Geometry: final body of the model. Coordinates: model frame, mm. A direction names the side the tool comes from. Coordinates: 2 decimals unless noted, no trailing zeros. Order: outer loops, then holes, each group sorted by start corner. A loop starts at its lowest first (then second) coordinate and runs counter-clockwise, first axis right, second up. Notation, with made-up numbers: (-39, 12.5) - (15, 12.5) arc R8 cw to (15, 20.5) - close; hole circle Ø8 at (16, -12). An arc over 180 degrees is marked (long way). Use a Markdown table: item, result. Add a question column.
```python
from build123d import *

# Parameters (mm, degrees)
SKETCH1_W                    = 83.185
SKETCH1_H                    = 41.91
SKETCH1_R                    = 2.54
SKETCH1_W_2                  = 57.15
SKETCH1_H_2                  = 25.4
ROVER_MOUNT_DEPTH            = 2.54
SIDE_WALLS_REACH             = 85.531
SIDE_WALLS_DIRECTION_2_DEPTH = 6.000000034
BACK_BRACES_DEPTH            = 2.54
FRONT_COVER_DEPTH            = 2.54
SKETCH5_W                    = 83.185
SKETCH5_H                    = 6.000000034
CLEANUP_DEPTH                = 31.75
FILLET1_R                    = 3.81
FILLET2_R                    = 6.35


with BuildPart() as part:
    # Sketch1 → Rover mount (new body)
    with BuildSketch(Plane.XY):
        with Locations((33.3375, -15.875)):
            Rectangle(SKETCH1_W, SKETCH1_H)
        with Locations((66.675, -31.75)):
            Circle(SKETCH1_R, mode=Mode.SUBTRACT)
        with Locations((69.85, 0)):
            Circle(SKETCH1_R, mode=Mode.SUBTRACT)
        with Locations((-3.175, -31.75)):
            Circle(SKETCH1_R, mode=Mode.SUBTRACT)
        Circle(SKETCH1_R, mode=Mode.SUBTRACT)
        with Locations((33.3375, -15.875)):
            Rectangle(SKETCH1_W_2, SKETCH1_H_2, mode=Mode.SUBTRACT)
    extrude(amount=ROVER_MOUNT_DEPTH)

    # Side Walls: up to this face of the body (flat: up to its plane)
    side_walls_end = Plane(part.part.faces().sort_by_distance((73.998539194, -15.875, 0))[0])
    # Sketch2 → Side Walls (add, up to the picked face)
    with BuildSketch(Plane.XY.offset(2.54), mode=Mode.PRIVATE) as side_walls_sk1:
        Polygon((-50.6625, -68.58), (-8.255, -68.58), (-8.255, -36.83), (4.445, -36.83), (4.445, -68.58), (62.23, -68.58), (62.23, -36.83), (74.93, -36.83), (74.93, -68.58), (117.3375, -68.58), (117.3375, 36.42), (122.4175, 36.42), (122.4175, -72.39), (-55.7425, -72.39), (-55.7425, 36.42), (-50.6625, 36.42), align=None)
    side_walls_tool1 = split(extrude(side_walls_sk1.sketch, amount=-SIDE_WALLS_REACH, mode=Mode.PRIVATE), bisect_by=side_walls_end, keep=Keep.BOTH, mode=Mode.PRIVATE)
    add(side_walls_tool1.solids().sort_by(Axis((-29.45875, -70.667597, 2.54), (0, 0, -1)))[0])

    # Sketch2 → Side Walls direction 2 (add)
    with BuildSketch(Plane.XY.offset(2.54)):
        Polygon((-50.6625, -68.58), (-8.255, -68.58), (-8.255, -36.83), (4.445, -36.83), (4.445, -68.58), (62.23, -68.58), (62.23, -36.83), (74.93, -36.83), (74.93, -68.58), (117.3375, -68.58), (117.3375, 36.42), (122.4175, 36.42), (122.4175, -72.39), (-55.7425, -72.39), (-55.7425, 36.42), (-50.6625, 36.42), align=None)
    extrude(amount=SIDE_WALLS_DIRECTION_2_DEPTH)

    # Sketch3 → Back Braces (add)
    with BuildSketch(Plane.XY.offset(2.54)):
        Polygon((-12.779899069, 1.716266635), (-55.7425, -68.58), (-49.3925, -68.58), (-8.255, -1.27), (-8.255, 5.08), (-55.7425, 36.42), (-55.7425, 30.07), align=None)
        Polygon((79.454899069, 1.716266635), (122.4175, -68.58), (116.0675, -68.58), (74.93, -1.27), (74.93, 5.08), (122.4175, 36.42), (122.4175, 30.07), align=None)
    extrude(amount=-BACK_BRACES_DEPTH)

    # Sketch4 → Front Cover (add)
    with BuildSketch(Plane.XY.offset(8.540000034)):
        Polygon((-55.7425, 36.42), (-45.5825, 36.42), (-45.5825, -63.5), (112.2575, -63.5), (112.2575, 36.42), (122.4175, 36.42), (122.4175, -72.39), (-55.7425, -72.39), align=None)
    extrude(amount=FRONT_COVER_DEPTH)

    # Sketch5 → Cleanup (cut)
    with BuildSketch(Plane(origin=(0, -36.83, 0), x_dir=(1, 0, 0), z_dir=(0, 1, 0))):
        with Locations((33.3375, -5.540000017)):
            Rectangle(SKETCH5_W, SKETCH5_H)
    extrude(amount=-CLEANUP_DEPTH, mode=Mode.SUBTRACT)

    # Fillet1
    fillet1_edges = [part.edges().sort_by_distance(p)[0] for p in [
        (117.3375, 26.717387207, 1.27),
        (117.3375, 33.067387207, 1.27),
        (117.3375, -60.268002431, 1.27),
        (79.454899069, 1.716266635, 1.27),
        (116.0675, -68.58, 1.27),
        (74.93, -1.27, 1.27),
        (-8.255, -68.58, 1.27),
        (4.445, -68.58, 1.27),
        (62.23, -68.58, 1.27),
        (74.93, -68.58, 1.27),
        (-8.255, 5.08, 1.27),
        (74.93, 5.08, 1.27),
        (-49.3925, -68.58, 1.27),
        (-12.779899069, 1.716266635, 1.27),
        (-50.6625, 33.067387207, 1.27),
        (-8.255, -1.27, 1.27),
        (-50.6625, -60.268002431, 1.27),
        (-50.6625, 26.717387207, 1.27),
    ]]
    fillet(fillet1_edges, radius=FILLET1_R)

    # Fillet2
    fillet2_edges = [part.edges().sort_by_distance(p)[0] for p in [
        (4.7625, -3.175, 1.27),
        (4.7625, -28.575, 1.27),
        (61.9125, -28.575, 1.27),
        (61.9125, -3.175, 1.27),
    ]]
    fillet(fillet2_edges, radius=FILLET2_R)


solid = part.part
```
1) Set-up query: faces 1 (the face through (34, -66, 8.54)), 2 (the face through (-45.95, -66.58, 1.25)), 3 (the face through (-30.797, -38.153, 1.288)). Return all of +Z, -Z, +X, -X, +Y, -Y with unobstructed straight access to the full face (end or side cutting, diameter ignored); none if empty.
2) Section B-B (x = 22.5). Return loops of the section in (y, z) (3 decimals), then the cut area to 3 significant figures.
3) Section D-D (y = -31.75). Give the number of separate pieces and of enclosed holes in the cut face, then the cut area to 3 significant figures.
4) Pin query (flat end, axial travel): pin 1 (2 mm diameter, centred on x = 40.5, z = 1.5, fed in from +Y); pin 2 (2.5 mm diameter, centred on x = -7.5, z = 5.5, fed in from +Y). Return the tip coordinate at first contact, or that it passes through.
5) Draft query along Z for faces 4 (the face through (95.48, 18.64, 1.29)), 5 (the face through (32, -68.58, 4)), 6 (the face through (47, -66, 11.08)). Return one class per face: pulls with the +Z half, pulls with the -Z half, needs draft (parallel to the pull), parting line crosses it, or undercut.
6) Ray query, line 1 along X through (y, z) = (-28, 4); line 2 along X through (y, z) = (-59, 9.5); line 3 along Y through (x, z) = (69.85, 0.95). Return the intervals inside material, ascending.
7) Section C-C (z = 4.75). Return loops of the section in (x, y), then the cut area to 3 significant figures.
8) Section A-A (y = -17.5). Return loops of the section in (x, z) (1 decimal).
Values follow:
| question | item | result |
|---|---|---|
| 1 | face 1 | +Y |
| 1 | face 2 | -Z |
| 1 | face 3 | +Z, -Z |
| 2 | outline | (-72.39, 0) - (-68.58, 0) - (-68.58, 8.54) - (-63.5, 8.54) - (-63.5, 11.08) - (-72.39, 11.08) - close; (-36.83, 0) - (-28.575, 0) - (-28.575, 2.54) - (-36.83, 2.54) - close; (-3.175, 0) - (5.08, 0) - (5.08, 2.54) - (-3.175, 2.54) - close |
| 2 | area | 97.1 mm² |
| 3 | separate pieces | 7 |
| 3 | enclosed holes | 0 |
| 3 | area | 356 mm² |
| 4 | pin 1 | stops at y = 5.08 |
| 4 | pin 2 | stops at y = -68.58 |
| 5 | face 4 | needs draft |
| 5 | face 5 | undercut |
| 5 | face 6 | pulls with the +Z half |
| 6 | line 1 | x = -55.74 to -50.66, 117.34 to 122.42 |
| 6 | line 2 | x = -55.74 to -45.58, 112.26 to 122.42 |
| 6 | line 3 | y = -72.39 to -2.54, 2.54 to 5.08 |
| 7 | outline | (-55.74, -72.39) - (122.42, -72.39) - (122.42, 36.42) - (117.34, 36.42) - (117.34, -68.58) - (-50.66, -68.58) - (-50.66, 36.42) - (-55.74, 36.42) - close |
| 7 | area | 1,750 mm² |
| 8 | outline | (-55.7, 0) - (-50.7, 0) - (-50.7, 8.5) - (-45.6, 8.5) - (-45.6, 11.1) - (-55.7, 11.1) - close; (-24.5, 0) - (-18.2, 0) - (-18.2, 2.5) - (-24.5, 2.5) - close; (-8.3, 0) - (4.8, 0) - (4.8, 2.5) - (-8.3, 2.5) - close; (61.9, 0) - (74.9, 0) - (74.9, 2.5) - (61.9, 2.5) - close; (84.8, 0) - (91.2, 0) - (91.2, 2.5) - (84.8, 2.5) - close; (112.3, 8.5) - (117.3, 8.5) - (117.3, 0) - (122.4, 0) - (122.4, 11.1) - (112.3, 11.1) - close |
